Autodesk Inventor part; units mm, degrees
ref_plane "YZ Plane" through (0, 0, 0) normal (1, 0, 0) x (0, 1, 0)
ref_plane "XZ Plane" through (0, 0, 0) normal (0, 1, 0) x (-1, 0, 0)
ref_plane "XY Plane" through (0, 0, 0) normal (0, 0, 1) x (1, 0, 0)
sketch "Sketch1" plane through (0, 0, 0) normal (0, 0, 1) x (1, 0, 0)
  circle A0 centre (-91.5, 0) radius 1.5
  circle A1 centre (91.5, 0) radius 1.5
  line L0 (0, -71.4835) -> (0, 99.0835) construction
  line L1 (95.5, 4) -> (95.5, -4)
  line L2 (93.5, -6) -> (-93.5, -6)
  line L3 (-95.5, -4) -> (-95.5, 4)
  line L4 (-207.6267, 0) -> (207.6267, 0) construction
  line L5 (-93.5, 6) -> (-95.5, 4)
  line L6 (-93.5, -6) -> (-95.5, -4)
  line L7 (95.5, -4) -> (93.5, -6)
  line L8 (93.5, 6) -> (95.5, 4)
  line L9 (-148.3048, 15) -> (148.3048, 15) construction
  circle A2 centre (-91.5, 30) radius 1.5
  circle A3 centre (91.5, 30) radius 1.5
  line L10 (0, 101.4835) -> (0, -69.0835)
  line L11 (95.5, 26) -> (95.5, 34)
  line L12 (93.5, 36) -> (-93.5, 36)
  line L13 (-95.5, 34) -> (-95.5, 26)
  line L14 (-93.5, 24) -> (-95.5, 26)
  line L15 (-93.5, 36) -> (-95.5, 34)
  line L16 (95.5, 34) -> (93.5, 36)
  line L17 (93.5, 24) -> (95.5, 26)
  line L18 (87.5822, -3.9178) -> (95.4178, 3.9178) construction
  line L19 (-83, 6) -> (-27.9101, 15)
  line L20 (0, 19.5597) -> (27.1798, 24)
  line L21 (83, 24) -> (27.9101, 15)
  line L22 (0, 10.4403) -> (-27.1798, 6)
  line L23 (83, 6) -> (27.9101, 15)
  line L24 (0, 19.5597) -> (-27.1798, 24)
  line L25 (-83, 24) -> (-27.9101, 15)
  line L26 (0, 10.4403) -> (27.1798, 6)
  line L27 (-93.5, 24) -> (-83, 24)
  line L28 (-93.5, 6) -> (-83, 6)
  line L29 (-27.1798, 6) -> (27.1798, 6)
  line L30 (83, 6) -> (93.5, 6)
  line L31 (-27.1798, 24) -> (27.1798, 24)
  line L32 (83, 24) -> (93.5, 24)
  point P0 (0, 0)
  point P1 (-95.5, 6)
  point P2 (95.5, -6)
  point P3 (95.5, 6)
  point P4 (-95.5, -6)
  point P5 (0, 30)
  point P6 (-95.5, 24)
  point P7 (95.5, 36)
  point P8 (95.5, 24)
  point P9 (-95.5, 36)
  dimension "d0" = 3
  dimension "d1" = 3
  dimension "d2" = 183
  dimension "d4" = 4
  dimension "d10" = 2
  dimension "d11" = 2
  dimension "d12" = 2
  dimension "d13" = 2
  dimension "d14" = 2
  dimension "d15" = 2
  dimension "d16" = 2
  dimension "d17" = 2
  dimension "d18" = 30
  dimension "d20" = 12
  dimension "d21" = 12
  dimension "d22" = 12
  dimension "d23" = 10.5
  dimension "d24" = 10.5
  dimension "d25" = 9
  dimension "d26" = 9
  dimension "d27" = 9
  dimension "d28" = 9
  dimension "d29" = 12
extrude "Extrusion2" add sketch "Sketch1" along normal blind 7.6 contours L1 L7 L2 L10 L29 L26 L20 L31 L12 L16 L11 L17 L32 L21 L23 L30 L8 | L2 L6 L3 L5 L28 L19 L25 L27 L14 L13 L15 L12 L10 L31 L24 L22 L29
sketch "Sketch2" plane through (-93.5, 36, 0) normal (0, 1, 0) x (1, 0, 0)
  line L0 (187, 0) -> (0, 0) construction
  line L1 (0, 0) -> (0, -7.6) construction
  line L2 (187, -7.6) -> (0, -7.6) construction
  line L3 (187, 0) -> (187, -7.6) construction
  line L4 (0, 0) -> (0, -7.6) construction
  line L5 (0, -3.8) -> (187, -3.8) construction
  line L6 (-2, -2) -> (15.5, -2)
  line L7 (15.5, -2) -> (15.5, -5.6)
  line L8 (15.5, -5.6) -> (-2, -5.6)
  line L9 (-2, -5.6) -> (-2, -2)
  line L10 (-2, 0) -> (-2, -7.6) construction
  line L11 (93.5, 0) -> (93.5, -7.6) construction
  line L12 (0, -7.6) -> (187, -7.6) construction
  line L13 (187, 0) -> (187, -7.6) construction
  line L14 (187, 0) -> (187, -7.6) construction
  line L15 (187, -3.8) -> (0, -3.8) construction
  line L16 (189, -2) -> (171.5, -2)
  line L17 (171.5, -2) -> (171.5, -5.6)
  line L18 (171.5, -5.6) -> (189, -5.6)
  line L19 (189, -5.6) -> (189, -2)
  line L20 (189, 0) -> (189, -7.6) construction
  dimension "d32" = 3.6
  dimension "d33" = 17.5
extrude "Extrusion3" cut sketch "Sketch2" against normal through all
properties part number "stabilizer"
Read the model definition and answer for the solid it produces. Units are mm, in the model's axes. A direction names the side the tool comes from. Round coordinates to 2 decimals unless told otherwise and drop trailing zeros. Write each loop counter-clockwise with the first axis right and the second up, starting at its lowest first coordinate (ties: lowest second). Pieces come first, ordered by that corner, then holes.
Q1. Flat-ended cylindrical pins translate along their axes: P1, Ø4, axis at x = 85.5, y = 32.5, coming from the -Z side; P2, Ø2.5, axis at x = 91.5, y = 0, coming from the -Z side. Find the tip coordinate at first contact, or state that the pin passes through.
Values:
P1: stops at z = 0
P2: passes through
Q2. A tool of negligible diameter and unlimited length cuts with its end or side. For faces 5 (the face through (-78, 30, 4)), 6 (the face through (92.306, 28.735, 0.986)), 7 (the face through (87, 30, 2)), from which of +Z, -Z, +X, -X, +Y, -Y can it reach the whole face along a straight path? Write none if from no direction.
Values:
face 5: -X, +Y, -Y
face 6: +Z, -Z
face 7: +X, +Y, -Y
Q3. Find section A-A on x = 31. Determine the outline of the cut face in (y, z), and give its area (3 significant figures).
Values:
outline: (-6, 0) - (14.5, 0) - (14.5, 7.6) - (-6, 7.6) - close; (15.5, 0) - (36, 0) - (36, 7.6) - (15.5, 7.6) - close
area: 312 mm2
Q4. The mould has two halves that part along Y. Classify faces 1 (the face through (1, 36, 4)), 2 (the face through (-1, 15, 7.6)), 3 (the face through (1, -6, 4)), 4 (the face through (55.841, 19.563, 3.747)): released by +Y, released by -Y, zero draft, split by the parting line, or undercut.
Values:
face 1: released by +Y
face 2: zero draft
face 3: released by -Y
face 4: undercut
Q5. Find section B-B on x = -60.5. Determine the outline of the cut face in (y, z).
Values:
outline: (-6, 0) - (9.68, 0) - (9.68, 7.6) - (-6, 7.6) - close; (20.32, 0) - (36, 0) - (36, 7.6) - (20.32, 7.6) - close
Q6. Straight lines are drawn through the part: line 1 (Y direction, x = -91.5, z = 6); line 2 (X direction, y = 0, z = 1.1); line 3 (Y direction, x = 25, z = 3). For each, find the intervals that lie inside material, in ascending order.
Values:
line 1: y = -6 to -1.5, 1.5 to 6, 24 to 28.5, 31.5 to 36
line 2: x = -95.5 to -93, -90 to 90, 93 to 95.5
line 3: y = -6 to 6, 6.36 to 23.64, 24 to 36
